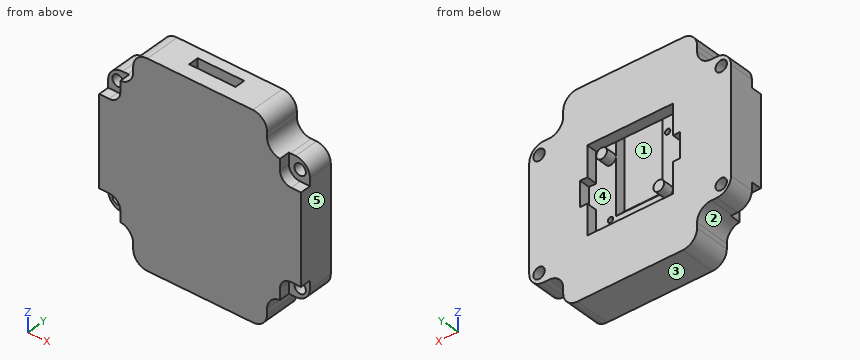
from build123d import *

# Parameters (mm, degrees)
AUFSATZ_LINEAR_AUSTRAGEN1_DEPTH      = 10
SKIZZE2_W                            = 24
SKIZZE2_H                            = 24
SCHNITT_LINEAR_AUSTRAGEN1_DEPTH      = 3
VERRUNDUNG1_R                        = 4
SKIZZE3_R                            = 1.5
AUFSATZ_LINEAR_AUSTRAGEN2_DEPTH      = 3
SKIZZE4_W                            = 2
SKIZZE4_H                            = 7
SCHNITT_LINEAR_AUSTRAGEN2_DEPTH      = 3
SKIZZE5_W                            = 13
SKIZZE5_H                            = 2.9
SCHNITT_LINEAR_AUSTRAGEN3_DEPTH      = 32
FASE1_SIZE                           = 4
F_3_2_3_2_DURCHMESSER_BOHRUNG1_D     = 3.2
F_3_2_3_2_DURCHMESSER_BOHRUNG1_DEPTH = 11
F_3_2_3_2_DURCHMESSER_BOHRUNG1_TIP   = 0.96137699
F_1_5_1_5_DURCHMESSER_BOHRUNG1_D     = 1.5
F_1_5_1_5_DURCHMESSER_BOHRUNG1_DEPTH = 5
F_1_5_1_5_DURCHMESSER_BOHRUNG1_TIP   = 0.450645464
SCHNITT_LINEAR_AUSTRAGEN4_DEPTH      = 3
SPIEGELN3_COPY_1_DEPTH               = 3


with BuildPart() as part:
    # Skizze1 → Aufsatz-Linear austragen1 (new body)
    with BuildSketch(Plane(origin=(0, 0, 0), x_dir=(1, 0, 0), z_dir=(0, 1, 0))):
        Polygon((18.75, 18.75), (28.25, 18.75), (28.25, -18.75), (18.75, -18.75), (18.75, -28.25), (-18.75, -28.25), (-18.75, -18.75), (-28.25, -18.75), (-28.25, 18.75), (-18.75, 18.75), (-18.75, 28.25), (18.75, 28.25), align=None)
    extrude(amount=AUFSATZ_LINEAR_AUSTRAGEN1_DEPTH)

    # Skizze2 → Schnitt-Linear austragen1 (cut)
    with BuildSketch(Plane(origin=(0, 10, 0), x_dir=(1, 0, 0), z_dir=(0, 1, 0))):
        Rectangle(SKIZZE2_W, SKIZZE2_H)
    extrude(amount=-SCHNITT_LINEAR_AUSTRAGEN1_DEPTH, mode=Mode.SUBTRACT)

    # Verrundung1
    verrundung1_edges = [part.edges().sort_by_distance(p)[0] for p in [
        (18.75, 5, 18.75),
        (18.75, 5, 28.25),
        (-18.75, 5, 28.25),
        (-18.75, 5, 18.75),
        (-28.25, 5, 18.75),
        (-28.25, 5, -18.75),
        (-18.75, 5, -18.75),
        (-18.75, 5, -28.25),
        (18.75, 5, -28.25),
        (18.75, 5, -18.75),
        (28.25, 5, -18.75),
        (28.25, 5, 18.75),
    ]]
    fillet(verrundung1_edges, radius=VERRUNDUNG1_R)

    # Skizze3 → Aufsatz-Linear austragen2 (add)
    with BuildSketch(Plane(origin=(0, 7, 0), x_dir=(1, 0, 0), z_dir=(0, 1, 0))):
        with Locations(Location((-8, 8, 0), (0, 0, 270))):
            Circle(SKIZZE3_R)
        with Locations(Location((8, -8, 0), (0, 0, 270))):
            Circle(SKIZZE3_R)
    extrude(amount=AUFSATZ_LINEAR_AUSTRAGEN2_DEPTH)

    # Skizze4 → Schnitt-Linear austragen2 (cut)
    with BuildSketch(Plane(origin=(0, 10, 0), x_dir=(1, 0, 0), z_dir=(0, 1, 0))):
        with Locations((13, 0)):
            Rectangle(SKIZZE4_W, SKIZZE4_H)
    schnitt_linear_austragen2 = extrude(amount=-SCHNITT_LINEAR_AUSTRAGEN2_DEPTH, mode=Mode.SUBTRACT)

    # Spiegeln1: Schnitt-Linear austragen2 across plane
    add(schnitt_linear_austragen2.mirror(Plane(origin=(0, 0, 0), x_dir=(0, 0, 1), z_dir=(1, 0, 0))), mode=Mode.SUBTRACT)

    # Skizze5 → Schnitt-Linear austragen3 (cut)
    with BuildSketch(Plane.XY.offset(28.25)):
        with Locations((0, 5.55)):
            Rectangle(SKIZZE5_W, SKIZZE5_H)
    extrude(amount=-SCHNITT_LINEAR_AUSTRAGEN3_DEPTH, mode=Mode.SUBTRACT)

    # Fase1
    # the kernel refuses this chamfer: 4 mm, written as the material it takes off along each edge
    with BuildSketch(Plane(origin=(-6.5, 7, -3.75), x_dir=(0, 0.027495876610586494, -0.9996219169112968), z_dir=(1, 0, 0))) as fase1_piece_1_section:
        Polygon((FASE1_SIZE * 0.999621916911, -FASE1_SIZE * 0.0274958766106), (-FASE1_SIZE * 0.0274958766106, -FASE1_SIZE * 0.999621916911), (0, 0), align=None)
    fase1_piece_1 = extrude(amount=13, mode=Mode.PRIVATE)
    fase1_piece_1 = split(fase1_piece_1, bisect_by=Plane(origin=(0, 4.1, -5.171489132), z_dir=(0, 1, 0)), keep=Keep.TOP, mode=Mode.PRIVATE)
    add(fase1_piece_1, mode=Mode.SUBTRACT)

    # Ø3.2 (3.2) Durchmesser Bohrung1
    with Locations(Plane(origin=(0, 10, 0), x_dir=(1, 0, 0), z_dir=(0, 1, 0))):
        with Locations((-25.5, -15.7), (25.5, 15.7), (25.5, -15.7), (-25.5, 15.7)):
            Hole(F_3_2_3_2_DURCHMESSER_BOHRUNG1_D / 2, depth=F_3_2_3_2_DURCHMESSER_BOHRUNG1_DEPTH)
            with Locations((0, 0, -(F_3_2_3_2_DURCHMESSER_BOHRUNG1_DEPTH + F_3_2_3_2_DURCHMESSER_BOHRUNG1_TIP / 2))):  # 118° drill point
                Cone(0, F_3_2_3_2_DURCHMESSER_BOHRUNG1_D / 2, F_3_2_3_2_DURCHMESSER_BOHRUNG1_TIP, mode=Mode.SUBTRACT)

    # Ø1.5 (1.5) Durchmesser Bohrung1
    with Locations(Plane(origin=(0, 7, 0), x_dir=(1, 0, 0), z_dir=(0, 1, 0))):
        with Locations((8, 8), (-8, -8)):
            Hole(F_1_5_1_5_DURCHMESSER_BOHRUNG1_D / 2, depth=F_1_5_1_5_DURCHMESSER_BOHRUNG1_DEPTH)
            with Locations((0, 0, -(F_1_5_1_5_DURCHMESSER_BOHRUNG1_DEPTH + F_1_5_1_5_DURCHMESSER_BOHRUNG1_TIP / 2))):  # 118° drill point
                Cone(0, F_1_5_1_5_DURCHMESSER_BOHRUNG1_D / 2, F_1_5_1_5_DURCHMESSER_BOHRUNG1_TIP, mode=Mode.SUBTRACT)

    # Skizze12 → Schnitt-Linear austragen4 (cut)
    with BuildSketch(Plane.XZ):
        with BuildLine():
            Line((-22.35, 15.7), (-22.35, 18.85))
            Line((-22.35, 18.85), (-25.5, 18.85))
            ThreePointArc((-25.5, 18.85), (-27.727386361, 17.927386361), (-28.65, 15.7))
            Line((-28.65, 15.7), (-28.65, 12.55))
            Line((-28.65, 12.55), (-25.5, 12.55))
            ThreePointArc((-25.5, 12.55), (-23.272613639, 13.472613639), (-22.35, 15.7))
        make_face()
    schnitt_linear_austragen4 = extrude(amount=-SCHNITT_LINEAR_AUSTRAGEN4_DEPTH, mode=Mode.SUBTRACT)

    # Spiegeln2: Schnitt-Linear austragen4 across plane
    add(schnitt_linear_austragen4.mirror(Plane(origin=(0, 0, 0), x_dir=(0, 0, 1), z_dir=(1, 0, 0))), mode=Mode.SUBTRACT)

    # Spiegeln3: Schnitt-Linear austragen4 across plane
    add(schnitt_linear_austragen4.mirror(Plane.XY), mode=Mode.SUBTRACT)

    # Spiegeln3 copy 1 sketch → Spiegeln3 copy 1 (cut)
    with BuildSketch(Plane(origin=(0, 0, 0), x_dir=(-1, 0, 0), z_dir=(0, -1, 0))):
        with BuildLine():
            Line((-22.35, 15.7), (-22.35, 18.85))
            Line((-22.35, 18.85), (-25.5, 18.85))
            ThreePointArc((-25.5, 18.85), (-27.727386361, 17.927386361), (-28.65, 15.7))
            Line((-28.65, 15.7), (-28.65, 12.55))
            Line((-28.65, 12.55), (-25.5, 12.55))
            ThreePointArc((-25.5, 12.55), (-23.272613639, 13.472613639), (-22.35, 15.7))
        make_face()
    extrude(amount=-SPIEGELN3_COPY_1_DEPTH, mode=Mode.SUBTRACT)


solid = part.part
The model under review builds one solid part; all positions refer to its coordinate system, in mm. Face numbers are marked on the shaded views. A direction names the side the tool comes from. Round coordinates to 2 decimals unless told otherwise and drop trailing zeros. Write each loop counter-clockwise with the first axis right and the second up, starting at its lowest first coordinate (ties: lowest second). Pieces come first, ordered by that corner, then holes. Notation, with made-up numbers: (2, 78) -> (34, 78) arc R8 cw to (34, 89) -> close; hole circle Ø8 at (16, 14.5). An arc over 180 degrees is marked (long way). Answer as a JSON object with one key per item and string values.
1. We need section A-A on x = -4.5. State the section outline as (y, z) points.
Results found:
{"outline": "(0, -28.25) -> (10, -28.25) -> (10, -12) -> (7, -12) -> (7, -7.75) -> (4.1, -4.85) -> (4.1, 28.25) -> (0, 28.25) -> close; (7, 12) -> (10, 12) -> (10, 28.25) -> (7, 28.25) -> close"}
2. To check wall thickness, follow line 1 along X through (y, z) = (5.25, 8); line 2 along X through (y, z) = (4.75, 0); line 3 along X through (y, z) = (6.5, -15.7). State the ranges of each line that lie inside material, in increasing order.
Results found:
{"line 1": "x = -28.25 to -8.75, -7.25 to -6.5, 6.5 to 28.25", "line 2": "x = -28.25 to -6.5, 6.5 to 28.25", "line 3": "x = -28.14 to -27.1, -23.9 to 23.9, 27.1 to 28.14"}
3. Machinability: for the marked faces 1 and 2, which of the approach directions +Z, -Z, +X, -X, +Y, -Y give a long, thin tool a straight path to every point of the face, cutting with its end or side? Answer none if there is none.
Results found:
{"face 1": "+Z", "face 2": "-Z, -X, +Y, -Y"}
4. We need section D-D on x = 20.5. State the section outline as (y, z) points.
Results found:
{"outline": "(0, -19.44) -> (10, -19.44) -> (10, 19.44) -> (0, 19.44) -> close"}
5. Clearance check with flat-ended pins moving along their axes: pin 1 (1.2 mm diameter, centred on x = -24, y = 8, fed in from +Z); pin 2 (0.8 mm diameter, centred on y = 7, z = -23.5, fed in from +X); pin 3 (5 mm diameter, centred on x = 25.5, z = -15.7, fed in from -Y). State where each tip first meets the part, or that it passes through.
Results found:
{"pin 1": "stops at z = 18.75", "pin 2": "stops at x = 18.75", "pin 3": "stops at y = 3"}
6. We need section B-B on y = 5. State how many separate pieces and enclosed holes the cut face has, and give its area (3 significant figures).
Results found:
{"separate pieces": "1", "enclosed holes": "6", "area": "2,340 mm^2"}
7. The part is to be moulded in two halves that separate along Z. For the marked faces 3, 4 and 5, say which applies: pulls with the +Z half, pulls with the -Z half, needs draft (parallel to the pull), parting line crosses it, or undercut.
Results found:
{"face 3": "pulls with the -Z half", "face 4": "undercut", "face 5": "needs draft"}
8. We need section C-C on z = 0.5. State the section outline as (x, y) points.
Results found:
{"outline": "(-28.25, 0) -> (28.25, 0) -> (28.25, 10) -> (14, 10) -> (14, 7) -> (6.5, 7) -> (6.5, 4.1) -> (-6.5, 4.1) -> (-6.5, 7) -> (-14, 7) -> (-14, 10) -> (-28.25, 10) -> close"}
